Autodesk Inventor part; units mm, degrees
ref_plane "YZ Plane" through (0, 0, 0) normal (1, 0, 0) x (0, 1, 0)
ref_plane "XZ Plane" through (0, 0, 0) normal (0, 1, 0) x (-1, 0, 0)
ref_plane "XY Plane" through (0, 0, 0) normal (0, 0, 1) x (1, 0, 0)
sketch "Boceto1" plane through (0, 0, 0) normal (0, 0, 1) x (1, 0, 0)
  line L0 (0, -12.2) -> (0, -206)
  line L1 (-3, -206) -> (-3, -12.2)
  line L2 (0, -206) -> (-3, -206)
  line L3 (-206, -203) -> (-206, 0)
  line L4 (-203, 0) -> (-203, -203)
  line L5 (-206, 0) -> (-203, 0)
  line L6 (-203, -203) -> (-3, -203)
  line L7 (-3, -203) -> (-3, -3)
  line L8 (-3, -3) -> (-203, -3)
  line L9 (-203, -3) -> (-203, -203)
  line L10 (-103, -203) -> (-103, -163)
  line L11 (-103, -163) -> (-143, -163)
  line L12 (-143, -163) -> (-63, -163)
  line L13 (-63, -163) -> (-63, -203)
  line L14 (-63, -203) -> (-143, -203)
  line L15 (-143, -203) -> (-143, -163)
  line L16 (-147.5, -3) -> (-147.5, -20.5)
  line L17 (-158.5, -20.5) -> (-158.5, -3)
  line L18 (-147.5, -3) -> (-147.5, -20.5)
  line L19 (-158.5, -3) -> (-147.5, -3)
  circle A0 centre (-191, -53) radius 2.1
  line L20 (-185.5, -58.5) -> (-203, -58.5)
  line L21 (-185.5, -47.5) -> (-185.5, -58.5)
  line L22 (-203, -47.5) -> (-185.5, -47.5)
  line L23 (-203, -58.5) -> (-203, -47.5)
  circle A1 centre (-53, -15) radius 2.1
  line L24 (-58.5, -20.5) -> (-58.5, -3)
  line L25 (-47.5, -20.5) -> (-58.5, -20.5)
  line L26 (-47.5, -3) -> (-47.5, -20.5)
  line L27 (-58.5, -3) -> (-47.5, -3)
  circle A2 centre (-15, -53) radius 2.1
  line L28 (-20.5, -47.5) -> (-3, -47.5)
  line L29 (-20.5, -58.5) -> (-20.5, -47.5)
  line L30 (-3, -58.5) -> (-20.5, -58.5)
  line L31 (-3, -47.5) -> (-3, -58.5)
  line L32 (-20.5, -147.5) -> (-3, -147.5)
  line L33 (-3, -158.5) -> (-20.5, -158.5)
  line L34 (-20.5, -158.5) -> (-20.5, -147.5)
  line L35 (-47.5, -185.5) -> (-47.5, -203)
  line L36 (-58.5, -203) -> (-58.5, -185.5)
  line L37 (-58.5, -185.5) -> (-47.5, -185.5)
  line L38 (-158.5, -203) -> (-158.5, -185.5)
  line L39 (-158.5, -185.5) -> (-147.5, -185.5)
  line L40 (-147.5, -185.5) -> (-147.5, -203)
  line L41 (-185.5, -158.5) -> (-203, -158.5)
  line L42 (-203, -147.5) -> (-185.5, -147.5)
  line L43 (-185.5, -147.5) -> (-185.5, -158.5)
  line L44 (-158.5, -3) -> (-147.5, -3)
  line L45 (-147.5, -3) -> (-147.5, -20.5)
  line L46 (-158.5, -20.5) -> (-158.5, -3)
  line L47 (-158.5, -3) -> (-147.5, -3)
  line L48 (-147.5, -3) -> (-147.5, -20.5)
  line L49 (-147.5, -20.5) -> (-158.5, -20.5)
  line L50 (-158.5, -20.5) -> (-158.5, -3)
  line L51 (-147.5, -22.5) -> (-160.5, -22.5)
  line L52 (-160.5, -22.5) -> (-160.5, -3)
  line L53 (-160.5, -3) -> (-145.5, -3)
  line L54 (-145.5, -3) -> (-145.5, -22.5)
  line L55 (-145.5, -22.5) -> (-160.5, -22.5)
  line L56 (-160.5, -22.5) -> (-160.5, -3)
  circle A3 centre (-103, -103) radius 47
  line L57 (-47.5, -22.5) -> (-60.5, -22.5)
  line L58 (-60.5, -22.5) -> (-60.5, -3)
  line L59 (-45.5, -3) -> (-45.5, -22.5)
  line L60 (-45.5, -22.5) -> (-60.5, -22.5)
  line L61 (-60.5, -22.5) -> (-60.5, -3)
  line L62 (-183.5, -160.5) -> (-203, -160.5)
  line L63 (-203, -147.5) -> (-185.5, -147.5)
  line L64 (-203, -147.5) -> (-185.5, -147.5)
  line L65 (-185.5, -158.5) -> (-203, -158.5)
  line L66 (-183.5, -160.5) -> (-203, -160.5)
  line L67 (-185.5, -158.5) -> (-203, -158.5)
  line L68 (-185.5, -158.5) -> (-203, -158.5)
  line L69 (-183.5, -147.5) -> (-183.5, -160.5)
  line L70 (-203, -147.5) -> (-185.5, -147.5)
  line L71 (-203, -147.5) -> (-185.5, -147.5)
  line L72 (-185.5, -147.5) -> (-185.5, -158.5)
  line L73 (-183.5, -145.5) -> (-183.5, -160.5)
  line L74 (-203, -145.5) -> (-183.5, -145.5)
  line L75 (-183.5, -47.5) -> (-183.5, -60.5)
  line L76 (-183.5, -45.5) -> (-183.5, -60.5)
  line L77 (-183.5, -60.5) -> (-203, -60.5)
  line L78 (-183.5, -60.5) -> (-203, -60.5)
  line L79 (-203, -45.5) -> (-183.5, -45.5)
  line L80 (-45.5, -183.5) -> (-45.5, -203)
  line L81 (-58.5, -203) -> (-58.5, -185.5)
  line L82 (-58.5, -203) -> (-58.5, -185.5)
  line L83 (-47.5, -185.5) -> (-47.5, -203)
  line L84 (-45.5, -183.5) -> (-45.5, -203)
  line L85 (-47.5, -185.5) -> (-47.5, -203)
  line L86 (-47.5, -185.5) -> (-47.5, -203)
  line L87 (-58.5, -183.5) -> (-45.5, -183.5)
  line L88 (-58.5, -203) -> (-58.5, -185.5)
  line L89 (-58.5, -203) -> (-58.5, -185.5)
  line L90 (-58.5, -185.5) -> (-47.5, -185.5)
  line L91 (-60.5, -183.5) -> (-45.5, -183.5)
  line L92 (-60.5, -203) -> (-60.5, -183.5)
  line L93 (-158.5, -183.5) -> (-145.5, -183.5)
  line L94 (-160.5, -183.5) -> (-145.5, -183.5)
  line L95 (-145.5, -183.5) -> (-145.5, -203)
  line L96 (-145.5, -183.5) -> (-145.5, -203)
  line L97 (-160.5, -203) -> (-160.5, -183.5)
  line L98 (-22.5, -45.5) -> (-3, -45.5)
  line L99 (-3, -58.5) -> (-20.5, -58.5)
  line L100 (-3, -58.5) -> (-20.5, -58.5)
  line L101 (-20.5, -47.5) -> (-3, -47.5)
  line L102 (-22.5, -45.5) -> (-3, -45.5)
  line L103 (-20.5, -47.5) -> (-3, -47.5)
  line L104 (-20.5, -47.5) -> (-3, -47.5)
  line L105 (-22.5, -58.5) -> (-22.5, -45.5)
  line L106 (-3, -58.5) -> (-20.5, -58.5)
  line L107 (-3, -58.5) -> (-20.5, -58.5)
  line L108 (-20.5, -58.5) -> (-20.5, -47.5)
  line L109 (-22.5, -60.5) -> (-22.5, -45.5)
  line L110 (-3, -60.5) -> (-22.5, -60.5)
  line L111 (-22.5, -158.5) -> (-22.5, -145.5)
  line L112 (-22.5, -160.5) -> (-22.5, -145.5)
  line L113 (-22.5, -145.5) -> (-3, -145.5)
  line L114 (-22.5, -145.5) -> (-3, -145.5)
  line L115 (-3, -160.5) -> (-22.5, -160.5)
  line L116 (-145.5, -183.5) -> (-60.5, -183.5)
  line L117 (-3, -3) -> (-18, -3)
  line L118 (-18, -3) -> (-18, -18)
  line L119 (-18, -18) -> (-3, -18)
  line L120 (-3, -18) -> (-3, -3)
  line L121 (-203, -3) -> (-188, -3)
  line L122 (-188, -3) -> (-188, -18)
  line L123 (-188, -18) -> (-203, -18)
  line L124 (-203, -18) -> (-203, -3)
  line L125 (-206, -203) -> (-203, -203)
  line L126 (0, -12.2) -> (-3, -12.2)
  point P0 (0, 0)
  point P1 (-3, -203)
  point P2 (-3, -160.5)
  point P3 (-3, -145.5)
  point P4 (-3, -60.5)
  point P5 (-3, -45.5)
  point P6 (-63, -183.5)
  point P7 (-143, -183.5)
  point P8 (-3, -18)
  dimension "d3" = 40
  dimension "d4" = 40
  dimension "d5" = 80
  dimension "d6" = 2
  dimension "d7" = 15
  dimension "d8" = 15
  dimension "d11" = 360
  dimension "d13" = 15
  dimension "d14" = 15
  dimension "d15" = 15
extrude "Extrusión1" add sketch "Boceto1" against normal blind 40 contours L1 L98 L105 L109 L110 L113 L111 L112 L115 L6 L80 L87 L91 L116 L13 L12 L11 L15 L93 L94 L97 L4 L62 L69 L73 L74 L77 L75 L76 L79 L123 L122 L8 L52 L51 L55 L54 L58 L57 L60 L59 L118 L119 | A3
shell "Vaciado1" thickness 0.8 removed faces 1 at (-103, -69.3333, -40)
properties part number "Contrapeso"
Can you work these out from the model? Positions are in its coordinate system, mm. A direction names the side the tool comes from. Give positions to 0.01 mm unless a question says otherwise; leave off trailing zeros. Loops run counter-clockwise (first coordinate to the right, second up) from the corner with the lowest first, then second, coordinate; pieces in that order, holes last. Notation, with made-up numbers: M 49,82.25 L 70,82.25 A11 ccw 70,86.25 Z; hole C 45.25,13.5 d3. An arc over 180 degrees is marked long. One line per item, written item: value.
(1) Will these pins go through, and if not, where does the flat tip stop? pin 1 (10 mm diameter, centred on y = -9.5, z = -24, fed in from -X); pin 2 (10 mm diameter, centred on y = -59, z = -15, fed in from -X); pin 3 (5 mm diameter, centred on x = -150.5, z = -28, fed in from +Y); pin 4 (6 mm diameter, centred on x = -194.5, z = -25, fed in from +Y).
Returned:
pin 1: x = -188
pin 2: x = -203
pin 3: y = -22.5
pin 4: y = -18
(2) Suppose I cut it at A-A on y = -117. List the corners of the cut face in (x, z) for me.
Returned:
outline: M -203,-40 L -202.2,-40 L -202.2,-0.8 L -3.8,-0.8 L -3.8,-40 L -3,-40 L -3,0 L -203,0 Z
(3) Which directions (+Z, -Z, +X, -X, +Y, -Y) give clear straight access to the entire face, cutting with the end or side of a thin tool? Please do faces 1 (the face through (-202.2, -181, -20)), 2 (the face through (-182, -203, -20)), 3 (the face through (-45.5, -193, -20)).
Returned:
face 1: -Z
face 2: +Z, -Z, +X, -X, -Y
face 3: +Z, -Z, -Y
(4) Suppose I cut it at B-B on x = -115.5. List the corners of the cut face in (y, z) for me.
Returned:
outline: M -163,-40 L -162.2,-40 L -162.2,-0.8 L -3.8,-0.8 L -3.8,-40 L -3,-40 L -3,0 L -163,0 Z
(5) I need wall thicknesses on line 1 (X direction, y = -14, z = -6.5); line 2 (Y direction, x = -13, z = -31.5); line 3 (X direction, y = -24.5, z = -19). Which ranges of each line are inside material? Lowest first, please.
Returned:
line 1: -188 to -187.2, -161.3 to -160.5, -145.5 to -144.7, -61.3 to -60.5, -45.5 to -44.7, -18.8 to -18
line 2: -203 to -202.2, -161.3 to -160.5, -145.5 to -144.7, -61.3 to -60.5, -45.5 to -44.7, -18.8 to -18
line 3: -203 to -202.2, -3.8 to -3
(6) We'd pull the mould along Y, two halves only. Please class faces 4 (the face through (-32, -3, -20)), 5 (the face through (-193, -160.5, -20)), 6 (the face through (-202.2, -32, -20)), 7 (the face through (-188, -10, -20)): released by +Y, released by -Y, zero draft, split by the parting line, or undercut.
Returned:
face 4: released by +Y
face 5: undercut
face 6: undercut
face 7: zero draft
